Could you check a few things on this model? Use its own coordinates, in mm. A direction names the side the tool comes from. Give positions to 0.01 mm unless a question says otherwise; leave off trailing zeros. Loops run counter-clockwise (first coordinate to the right, second up) from the corner with the lowest first, then second, coordinate; pieces in that order, holes last. Notation, with made-up numbers: (84.25, 85) -> (140.25, 85) arc R32 ccw to (140.25, 123) -> close; hole circle Ø4 at (12.5, 36). An arc over 180 degrees is marked (long way). Put each result on its own line as item: value.
```python
from build123d import *

# Parameters (mm, degrees)
BOSS_EXTRUDE1_DEPTH                = 9.525
F_1_4_20_TAPPED_HOLE1_D            = 5.1054
F_5_16_0_3125_DIAMETER_HOLE1_D     = 7.9375
F_5_16_0_3125_DIAMETER_HOLE1_DEPTH = 20.6365
F_1_4_20_TAPPED_HOLE2_D            = 5.1054
F_1_4_20_TAPPED_HOLE2_DEPTH        = 16.51
F_1_4_20_TAPPED_HOLE2_TIP          = 1.533816902


with BuildPart() as part:
    # Sketch3 → Boss-Extrude1 (new, symmetric)
    with BuildSketch(Plane(origin=(0, 0, 0), x_dir=(0, 0, -1), z_dir=(1, 0, 0))):
        Polygon((-53.975, 14.2875), (-53.975, -17.4625), (9.525, -17.4625), (9.525, -6.35), (-34.925, -6.35), (-34.925, 6.35), (9.525, 6.35), (9.525, 14.2875), align=None)
    extrude(amount=BOSS_EXTRUDE1_DEPTH, both=True)

    # 1/4-20 Tapped Hole1 (through all)
    with Locations(Plane(origin=(0, 14.2875, 0), x_dir=(1, 0, 0), z_dir=(0, 1, 0))):
        with Locations((0, 0)):
            Hole(F_1_4_20_TAPPED_HOLE1_D / 2)

    # 5/16 (0.3125) Diameter Hole1
    with Locations(Plane(origin=(0, 14.2875, 0), x_dir=(1, 0, 0), z_dir=(0, 1, 0))):
        with Locations((0, 0)):
            Hole(F_5_16_0_3125_DIAMETER_HOLE1_D / 2, depth=F_5_16_0_3125_DIAMETER_HOLE1_DEPTH)

    # 1/4-20 Tapped Hole2
    with Locations(Plane.XY.offset(53.975)):
        with Locations((0, -12.7)):
            Hole(F_1_4_20_TAPPED_HOLE2_D / 2, depth=F_1_4_20_TAPPED_HOLE2_DEPTH)
            with Locations((0, 0, -(F_1_4_20_TAPPED_HOLE2_DEPTH + F_1_4_20_TAPPED_HOLE2_TIP / 2))):  # 118° drill point
                Cone(0, F_1_4_20_TAPPED_HOLE2_D / 2, F_1_4_20_TAPPED_HOLE2_TIP, mode=Mode.SUBTRACT)


solid = part.part
```
1. I need wall thicknesses on line 1 (Z direction, x = 0.25, y = 12.5) (3 decimals); line 2 (Y direction, x = 3.5, z = 17.5); line 3 (Z direction, x = 0, y = -9.75) (3 decimals). Which ranges of each line are inside material? Lowest first, please.
Recorded:
line 1: z = -9.525 to -3.961, 3.961 to 53.975
line 2: y = -17.46 to -6.35, 6.35 to 14.29
line 3: z = -9.525 to -2.553, 2.553 to 53.975
2. For faces 1 (the face through (0, 0, 34.925)), 2 (the face through (0.553, -15.192, 45.604)), 3 (the face through (0.86, 10.263, 3.874)), which set-ups out of +Z, -Z, +X, -X, +Y, -Y let a thin tool reach every point of the face, with its end or its side?
Recorded:
face 1: -Z, +X, -X
face 2: +Z
face 3: +Y
3. If we section it at A-A (z = 0): Count the separate pieces of the cut face and the enclosed holes in it, then the cut area to 3 significant figures.
Recorded:
separate pieces: 4
enclosed holes: 0
area: 243 mm^2
4. If we section it at C-C (y = -9): List the corners of the cut face in (x, z) for me (3 decimals).
Recorded:
outline: (-9.525, -9.525) -> (9.525, -9.525) -> (9.525, 53.975) -> (-9.525, 53.975) -> close; hole circle Ø5.105 at (0, 0)
5. I'm going to push flat-ended pins straight in: pin 1 (6.5 mm diameter, centred on x = 0, z = 0, fed in from +Y); pin 2 (4.5 mm diameter, centred on x = 0, y = -12.7, fed in from +Z); pin 3 (6.5 mm diameter, centred on x = 4, y = 0.5, fed in from -Z) (3 decimals); pin 4 (5 mm diameter, centred on x = 0, z = 0, fed in from -Y). Where does each tip first touch, or does it pass through?
Recorded:
pin 1: stops at y = -6.35
pin 2: stops at z = 37.28
pin 3: stops at z = 34.925
pin 4: passes through
6. Thinking about a two-plate mould opening in Y: for faces 4 (the face through (0, 6.35, 13)), 5 (the face through (0, 14.288, 22)), 6 (the face through (-2.435, -11.984, -0.767)), 7 (the face through (0, -17.462, 23)), which applies, pulls with the +Y half, pulls with the -Y half, needs draft (parallel to the pull), parting line crosses it, or undercut?
Recorded:
face 4: undercut
face 5: pulls with the +Y half
face 6: needs draft
face 7: pulls with the -Y half
